The drawing under review shows one solid part. Ordinate dimensions are in mm from its lowest x, y, z. A direction names the side the tool comes from. Give positions to 0.01 mm unless a question says otherwise; leave off trailing zeros. Loops run counter-clockwise (first coordinate to the right, second up) from the corner with the lowest first, then second, coordinate; pieces in that order, holes last. Notation, with made-up numbers: M -9.75,4 L 20.25,4 A29 cw 20.25,40 Z; hole C 46.25,16.5 d1. An arc over 180 degrees is marked long. Write item = value, one per line. Start each with the question number.
1. Draft analysis for pull direction Z (two halves, no side actions). For the marked faces 4, 5 and 6, state which applies: pulls with the +Z half, pulls with the -Z half, needs draft (parallel to the pull), parting line crosses it, or undercut.
2. We need section A-A on y = 35.5. Give the boundary of the cut face in (x, z), then the cut area to 3 significant figures.
3. For the marked faces 1, 2 and 3, list the 3-axis set-ups (+Z, -Z, +X, -X, +Y, -Y) from which the entire face can be reached by the end or side of a thin tool; tool diameter is ignored.
4. For pin 1 (5.5 mm diameter, centred on x = 22.5, z = 42.5, fed in from -Y); pin 2 (6 mm diameter, centred on x = 23.5, z = 27.5, fed in from +Y); pin 3 (8 mm diameter, centred on x = 18, z = 12.5, fed in from +Y), all flat-tipped, find the tip position at first contact; note any pin that passes through.
5. We need section C-C on x = 33. Give the boundary of the cut face in (y, z), then the cut area to 3 significant figures.
6. We need section B-B on z = 45. Give the boundary of the cut face in (x, y).
7. We need section D-D on z = 13. Give the boundary of the cut face in (x, y).
8. Wall thickness on line 1 along Y through (x, z) = (23.5, 55.5); line 2 along Y through (x, z) = (6, 44); line 3 along X through (y, z) = (3.5, 50.5): over which ranges is each line inside the solid? List them lowest first. Write a range as from..to.
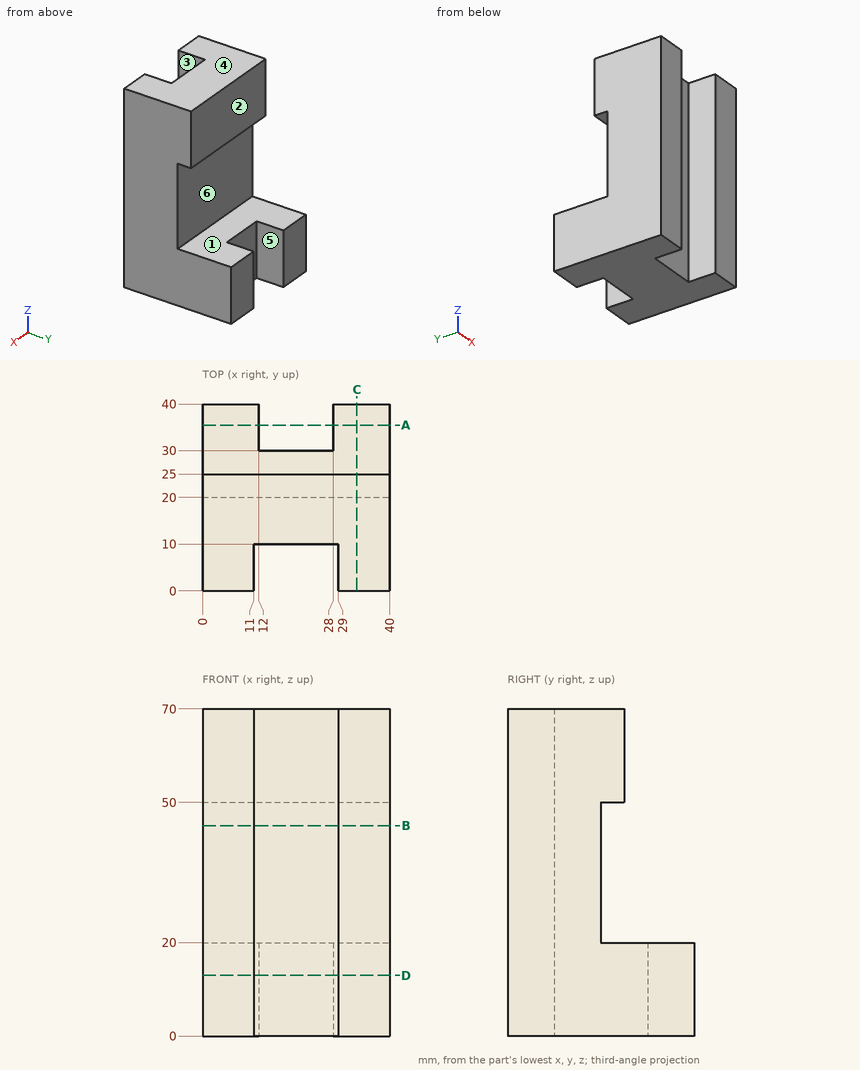
Final values:
q1.face_4 = pulls with the +Z half
q1.face_5 = needs draft
q1.face_6 = undercut
q2.outline = M 0,0 L 12,0 L 12,20 L 0,20 Z; M 28,0 L 40,0 L 40,20 L 28,20 Z
q2.area = 480 mm²
q3.face_1 = +X, -X, +Y
q3.face_2 = +Z, +X, -X, +Y
q3.face_3 = +Z, -Z, -Y
q4.pin_1 = 10
q4.pin_2 = 20
q4.pin_3 = 30
q5.outline = M 0,0 L 40,0 L 40,20 L 20,20 L 20,50 L 25,50 L 25,70 L 0,70 Z
q5.area = 1,900 mm²
q6.outline = M 0,0 L 11,0 L 11,10 L 29,10 L 29,0 L 40,0 L 40,20 L 0,20 Z
q7.outline = M 0,0 L 11,0 L 11,10 L 29,10 L 29,0 L 40,0 L 40,40 L 28,40 L 28,30 L 12,30 L 12,40 L 0,40 Z
q8.line_1 = 10..25
q8.line_2 = 0..20
q8.line_3 = 0..11, 29..40
